```python
from build123d import *

# Parameters (mm, degrees)
SKETCH_1_R          = 7.5
EXTRUDE_1_DEPTH     = 18.5
SKETCH_2_R          = 1.5
EXTRUDE_2_DEPTH     = 10
SKETCH_3_R          = 1
CUT_EXTRUDE_1_DEPTH = 10


with BuildPart() as part:
    # 草图1 → 凸台-拉伸1 (new body)
    with BuildSketch(Plane(origin=(0, 0, 0), x_dir=(1, 0, 0), z_dir=(0, 1, 0))):
        with Locations(Location((0, 0, 0), (0, 0, 270))):
            Circle(SKETCH_1_R)
    extrude(amount=EXTRUDE_1_DEPTH)

    # 草图2 → 凸台-拉伸2 (add)
    with BuildSketch(Plane(origin=(0, 18.5, 0), x_dir=(1, 0, 0), z_dir=(0, 1, 0))):
        with Locations(Location((0, 0, 0), (0, 0, 270))):
            Circle(SKETCH_2_R)
    extrude(amount=EXTRUDE_2_DEPTH)

    # 草图3 → 切除-拉伸1 (cut)
    with BuildSketch(Plane(origin=(0, 18.5, 0), x_dir=(1, 0, 0), z_dir=(0, 1, 0))):
        with Locations(Location((-5.5, 0, 0), (0, 0, 270))):
            Circle(SKETCH_3_R)
        with Locations(Location((5.5, 0, 0), (0, 0, 270))):
            Circle(SKETCH_3_R)
    extrude(amount=-CUT_EXTRUDE_1_DEPTH, mode=Mode.SUBTRACT)


solid = part.part
```
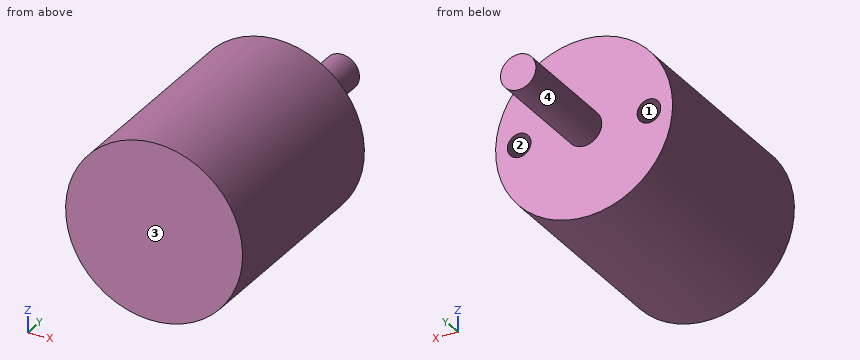
Can you work these out from the model? Positions are in its coordinate system, mm. Face numbers are marked on the shaded views. Give positions to 0.01 mm unless a question says otherwise; leave off trailing zeros. Write each loop counter-clockwise with the first axis right and the second up, starting at its lowest first coordinate (ties: lowest second). Pieces come first, ordered by that corner, then holes. Notation, with made-up numbers: (58.25, 75) -> (99.25, 75) arc R23 cw to (99.25, 106) -> close; hole circle Ø1 at (75.5, -0.75). An arc over 180 degrees is marked (long way). Write item = value, one per line.
(1) Suppose I cut it at D-D on y = 20.5. Write out the boundary of the cut face in (x, z).
Worked out:
outline = circle Ø3 at (0, 0)
(2) I'm going to push flat-ended pins straight in: P1, Ø1.5, axis at y = 18.5, z = 3.5, coming from the +X side; P2, Ø2, axis at y = 11, z = -3, coming from the +X side; P3, Ø5, axis at x = -4.5, z = -2, coming from the +Y side. Where does each tip first touch, or does it pass through?
Worked out:
P1 = 6.98
P2 = 7.23
P3 = 18.5
(3) Thinking about a two-plate mould opening in X: for the marked faces 1, 2, 3 and 4, which applies, released by +X, released by -X, zero draft, split by the parting line, or undercut?
Worked out:
face_1 = undercut
face_2 = undercut
face_3 = zero draft
face_4 = split by the parting line
(4) I need wall thicknesses on probe 1 along X at (y, z) = (14, 0); probe 2 along Y at (x, z) = (-0.5, 2.25); probe 3 along Z at (x, y) = (-0.25, 3.5). Which ranges of each line are inside material? Lowest first, please. Write a range as from..to.
Worked out:
probe_1 = -7.5..-6.5, -4.5..4.5, 6.5..7.5
probe_2 = 0..18.5
probe_3 = -7.5..7.5
(5) Suppose I cut it at C-C on x = 5.5. Write out the boundary of the cut face in (y, z).
Worked out:
outline = (0, -5.1) -> (18.5, -5.1) -> (18.5, -1) -> (8.5, -1) -> (8.5, 1) -> (18.5, 1) -> (18.5, 5.1) -> (0, 5.1) -> close
(6) Suppose I cut it at A-A on y = 14.5. Write out the boundary of the cut face in (x, z), then the cut area to 3 significant figures.
Worked out:
outline = circle Ø15 at (0, 0); hole circle Ø2 at (-5.5, 0); hole circle Ø2 at (5.5, 0)
area = 170 mm^2
(7) Suppose I cut it at B-B on z = 0. Write out the boundary of the cut face in (x, y).
Worked out:
outline = (-7.5, 0) -> (7.5, 0) -> (7.5, 18.5) -> (6.5, 18.5) -> (6.5, 8.5) -> (4.5, 8.5) -> (4.5, 18.5) -> (1.5, 18.5) -> (1.5, 28.5) -> (-1.5, 28.5) -> (-1.5, 18.5) -> (-4.5, 18.5) -> (-4.5, 8.5) -> (-6.5, 8.5) -> (-6.5, 18.5) -> (-7.5, 18.5) -> close
